Verification items for the finished model (mm, model axes). Give positions to 0.01 mm unless a question says otherwise; leave off trailing zeros. Write each loop counter-clockwise with the first axis right and the second up, starting at its lowest first coordinate (ties: lowest second). Pieces come first, ordered by that corner, then holes. Notation, with made-up numbers: (72, -14) -> (93, -14) arc R11 cw to (93, -3) -> close; hole circle Ø6 at (55, 55). An arc over 180 degrees is marked (long way). Write item = value, one per line.
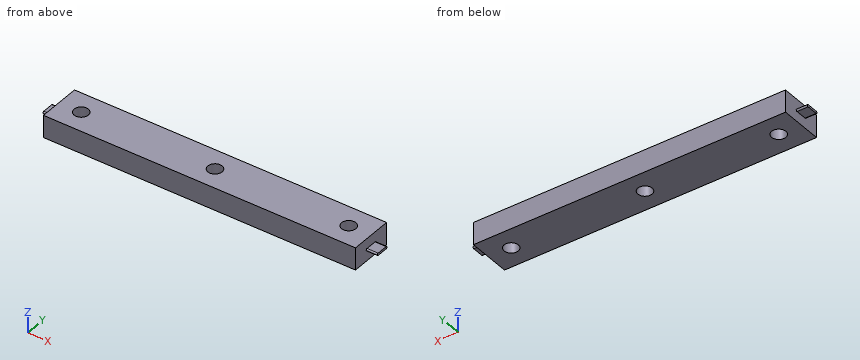
from build123d import *

# Parameters (mm, degrees)
SKETCH1_W           = 177.8
SKETCH1_H           = 24.555331286
SKETCH1_R           = 4.064
BOSS_EXTRUDE1_DEPTH = 12.7
BOSS_EXTRUDE2_DEPTH = 6.35
BOSS_EXTRUDE3_START = 6.35
BOSS_EXTRUDE3_DEPTH = 6.35


with BuildPart() as part:
    # Sketch1 → Boss-Extrude1 (new body)
    with BuildSketch(Plane.XY):
        Rectangle(SKETCH1_W, SKETCH1_H)
        Circle(SKETCH1_R, mode=Mode.SUBTRACT)
        with Locations((-76.2, 0)):
            Circle(SKETCH1_R, mode=Mode.SUBTRACT)
        with Locations((76.2, 0)):
            Circle(SKETCH1_R, mode=Mode.SUBTRACT)
    extrude(amount=BOSS_EXTRUDE1_DEPTH)

    # Sketch2 → Boss-Extrude2 (add)
    with BuildSketch(Plane.ZY.offset(88.9)):
        with BuildLine():
            Line((5.715, -3.175), (5.715, 3.175))
            ThreePointArc((5.715, 3.175), (6.35, 3.81), (6.985, 3.175))
            Line((6.985, 3.175), (6.985, -3.175))
            ThreePointArc((6.985, -3.175), (6.35, -3.81), (5.715, -3.175))
        make_face()
    extrude(amount=BOSS_EXTRUDE2_DEPTH)

    # Sketch3 → Boss-Extrude3 (add)
    with BuildSketch(Plane(origin=(88.9, 0, 0), x_dir=(0, 0, -1), z_dir=(1, 0, 0)).offset(BOSS_EXTRUDE3_START)):
        with BuildLine():
            Line((-5.715, 3.175), (-5.715, -3.175))
            ThreePointArc((-5.715, -3.175), (-6.35, -3.81), (-6.985, -3.175))
            Line((-6.985, -3.175), (-6.985, 3.175))
            ThreePointArc((-6.985, 3.175), (-6.35, 3.81), (-5.715, 3.175))
        make_face()
    extrude(amount=-BOSS_EXTRUDE3_DEPTH)


solid = part.part
Item 1: Sectioned sample at D-D on y = -8.75. Record the cut outline in (x, z), then the cut area to 3 significant figures.
Response values:
outline = (-88.9, 0) -> (88.9, 0) -> (88.9, 12.7) -> (-88.9, 12.7) -> close
area = 2,260 mm^2
Item 2: Sectioned sample at B-B on y = 0. Record the cut outline in (x, z) (3 decimals), then the cut area to 3 significant figures.
Response values:
outline = (-95.25, 5.715) -> (-88.9, 5.715) -> (-88.9, 0) -> (-80.264, 0) -> (-80.264, 12.7) -> (-88.9, 12.7) -> (-88.9, 6.985) -> (-95.25, 6.985) -> close; (-72.136, 0) -> (-4.064, 0) -> (-4.064, 12.7) -> (-72.136, 12.7) -> close; (4.064, 0) -> (72.136, 0) -> (72.136, 12.7) -> (4.064, 12.7) -> close; (80.264, 0) -> (88.9, 0) -> (88.9, 5.715) -> (95.25, 5.715) -> (95.25, 6.985) -> (88.9, 6.985) -> (88.9, 12.7) -> (80.264, 12.7) -> close
area = 1,960 mm^2
Item 3: Material ranges on line 1 (Y direction, x = 76.2, z = 8.25); line 2 (X direction, y = 3.5, z = 6.5); line 3 (X direction, y = 3.75, z = 5), recorded low to high.
Response values:
line_1 = -12.28 to -4.06, 4.06 to 12.28
line_2 = -95.25 to -78.27, -74.13 to -2.07, 2.07 to 74.13, 78.27 to 95.25
line_3 = -88.9 to -77.77, -74.63 to -1.57, 1.57 to 74.63, 77.77 to 88.9
Item 4: Sectioned sample at C-C on x = 76.2. Record the cut outline in (y, z).
Response values:
outline = (-12.28, 0) -> (-4.06, 0) -> (-4.06, 12.7) -> (-12.28, 12.7) -> close; (4.06, 0) -> (12.28, 0) -> (12.28, 12.7) -> (4.06, 12.7) -> close
Item 5: Sectioned sample at A-A on z = 2.5. Record the cut outline in (x, y).
Response values:
outline = (-88.9, -12.28) -> (88.9, -12.28) -> (88.9, 12.28) -> (-88.9, 12.28) -> close; hole circle Ø8.13 at (-76.2, 0); hole circle Ø8.13 at (0, 0); hole circle Ø8.13 at (76.2, 0)
Item 6: Go/stop test with flat-tipped pins: P1, Ø5, axis at x = -91.5, y = 0, coming from the -Z side (3 decimals); P2, Ø13, axis at x = -76.2, y = 0, coming from the +Z side; P3, Ø7, axis at x = 93.5, y = 0, coming from the +Z side (3 decimals); P4, Ø2, axis at y = -4, z = 9, coming from the -X side. Record where each tip stops, or that it passes through.
Response values:
P1 = 5.715
P2 = 12.7
P3 = 6.985
P4 = -88.9
